```python
from build123d import *

# Parameters (mm, degrees)
BOSS_EXTRUDE1_DEPTH = 4


with BuildPart() as part:
    # Sketch1 → Boss-Extrude1 (new body)
    with BuildSketch(Plane(origin=(-22.493180964, 0, 0), x_dir=(0, 0, -1), z_dir=(1, 0, 0))):
        with BuildLine():
            Line((41.499999434, -352.52261402), (41.499999434, 26.477385891))
            ThreePointArc((41.499999434, 26.477385891), (40.914212996, 27.891599453), (39.499999434, 28.477385891))
            Line((39.499999434, 28.477385891), (-359.500000477, 28.477385891))
            ThreePointArc((-359.500000477, 28.477385891), (-360.914214039, 27.891599453), (-361.500000477, 26.477385891))
            Line((-361.500000477, 26.477385891), (-361.500000477, -87.499667694))
            ThreePointArc((-361.500000477, -87.499667694), (-360.914214039, -88.913881256), (-359.500000477, -89.499667694))
            Line((-359.500000477, -89.499667694), (-322.5, -89.499667694))
            ThreePointArc((-322.5, -89.499667694), (-320.025126266, -90.524793959), (-319, -92.999667694))
            Line((-319, -92.999667694), (-319, -232.999667694))
            ThreePointArc((-319, -232.999667694), (-320.025126266, -235.474541428), (-322.5, -236.499667694))
            Line((-322.5, -236.499667694), (-359.500000477, -236.499667694))
            ThreePointArc((-359.500000477, -236.499667694), (-360.914214039, -237.085454131), (-361.500000477, -238.499667694))
            Line((-361.500000477, -238.499667694), (-361.500000477, -352.52261402))
            ThreePointArc((-361.500000477, -352.52261402), (-360.914214039, -353.936827582), (-359.500000477, -354.52261402))
            Line((-359.500000477, -354.52261402), (39.499999434, -354.52261402))
            ThreePointArc((39.499999434, -354.52261402), (40.914212996, -353.936827582), (41.499999434, -352.52261402))
        make_face()
    extrude(amount=-BOSS_EXTRUDE1_DEPTH)


solid = part.part
```
Verification items for the finished model (mm, model axes). Coordinates: 2 decimals unless noted, no trailing zeros. Write each loop counter-clockwise with the first axis right and the second up, starting at its lowest first coordinate (ties: lowest second). Pieces come first, ordered by that corner, then holes. Notation, with made-up numbers: M -21,13.5 L 26,13.5 A30 ccw 26,50.5 Z; hole C 22,27.5 d11. An arc over 180 degrees is marked long. One line per item, written item: value.
Item 1: Section check B-B, the plane x = -23.2. Record the boundary of the cut face in (y, z), plus the area to 3 significant figures.
Check sheet entries:
outline: M -354.52,-39.5 A2 ccw -352.52,-41.5 L 26.48,-41.5 A2 ccw 28.48,-39.5 L 28.48,359.5 A2 ccw 26.48,361.5 L -87.5,361.5 A2 ccw -89.5,359.5 L -89.5,322.5 A3.5 cw -93,319 L -233,319 A3.5 cw -236.5,322.5 L -236.5,359.5 A2 ccw -238.5,361.5 L -352.52,361.5 A2 ccw -354.52,359.5 Z
area: 148,000 mm^2
Item 2: Section check A-A, the plane z = 327. Record the boundary of the cut face in (x, y), plus the area to 3 significant figures.
Check sheet entries:
outline: M -26.49,-354.52 L -22.49,-354.52 L -22.49,-236.5 L -26.49,-236.5 Z; M -26.49,-89.5 L -22.49,-89.5 L -22.49,28.48 L -26.49,28.48 Z
area: 944 mm^2
Item 3: Scan line: line 1 along Z through (x, y) = (-26.3, -124). Record every from-to range of solid material in increasing order.
Check sheet entries:
line 1: z = -41.5 to 319
Item 4: Gauge pin test, flat end, axial feed: pin 1 Ø2 at (x, y) = (-24, -143) entering from +Z. Record the tip position at first contact, or that the pin passes through.
Check sheet entries:
pin 1: stops at z = 319
Item 5: Section check C-C, the plane y = -124. Record the boundary of the cut face in (x, z), plus the area to 3 significant figures.
Check sheet entries:
outline: M -26.49,-41.5 L -22.49,-41.5 L -22.49,319 L -26.49,319 Z
area: 1,440 mm^2
